CAD build for the part. Positions are in the model's coordinates, mm. A direction names the side the tool comes from. Give positions to 0.01 mm unless a question says otherwise; leave off trailing zeros. Loops run counter-clockwise (first coordinate to the right, second up) from the corner with the lowest first, then second, coordinate; pieces in that order, holes last. Notation, with made-up numbers: M 51,39.25 L 84,39.25 A23 cw 84,67.25 Z; hole C 86,27 d1. An arc over 180 degrees is marked long. One line per question, with ' | ' between items.
```python
from build123d import *

# Parameters (mm, degrees)
SKETCH1_W           = 40.64
SKETCH1_H           = 47.625
SKETCH1_R           = 3.048
BOSS_EXTRUDE1_DEPTH = 6.35
BOSS_EXTRUDE2_DEPTH = 9.906
SKETCH3_R           = 4.826
CUT_EXTRUDE1_DEPTH  = 76.04657711
SKETCH4_R           = 7.1374
CUT_EXTRUDE2_DEPTH  = 9.906
CHAMFER1_SIZE       = 1.5875


with BuildPart() as part:
    # Sketch1 → Boss-Extrude1 (new body)
    with BuildSketch(Plane(origin=(0, 0, 0), x_dir=(1, 0, 0), z_dir=(0, 1, 0))):
        with Locations((20.32, 37.1475)):
            Rectangle(SKETCH1_W, SKETCH1_H)
        with Locations(Location((30.987358569, 18.161641431, 0), (0, 0, 270))):
            Circle(SKETCH1_R, mode=Mode.SUBTRACT)
        with Locations(Location((30.987358569, 43.306358569, 0), (0, 0, 270))):
            Circle(SKETCH1_R, mode=Mode.SUBTRACT)
        with Locations(Location((5.842641431, 18.161641431, 0), (0, 0, 270))):
            Circle(SKETCH1_R, mode=Mode.SUBTRACT)
        with Locations(Location((5.842641431, 43.306358569, 0), (0, 0, 270))):
            Circle(SKETCH1_R, mode=Mode.SUBTRACT)
    extrude(amount=BOSS_EXTRUDE1_DEPTH)

    # Sketch2 → Boss-Extrude2 (add)
    with BuildSketch(Plane(origin=(0, 6.35, 0), x_dir=(1, 0, 0), z_dir=(0, 1, 0))):
        Polygon((31.115, 30.734), (24.765, 41.732522628), (12.065, 41.732522628), (5.715, 30.734), (12.065, 19.735477372), (24.765, 19.735477372), align=None)
    extrude(amount=BOSS_EXTRUDE2_DEPTH)

    # Sketch3 → Cut-Extrude1 (cut, through all)
    with BuildSketch(Plane(origin=(0, 16.256, 0), x_dir=(1, 0, 0), z_dir=(0, 1, 0))):
        with Locations(Location((18.415, 30.734, 0), (0, 0, 270))):
            Circle(SKETCH3_R)
    extrude(amount=-CUT_EXTRUDE1_DEPTH, mode=Mode.SUBTRACT)

    # Sketch4 → Cut-Extrude2 (cut)
    with BuildSketch(Plane(origin=(0, 16.256, 0), x_dir=(1, 0, 0), z_dir=(0, 1, 0))):
        with Locations(Location((18.415, 30.734, 0), (0, 0, 270))):
            Circle(SKETCH4_R)
    extrude(amount=-CUT_EXTRUDE2_DEPTH, mode=Mode.SUBTRACT)

    # Chamfer1
    chamfer1_edges = [part.edges().sort_by_distance(p)[0] for p in [
        (20.32, 6.35, -60.96),
        (0, 6.35, -37.1475),
        (27.94, 16.256, -25.234738686),
        (27.94, 16.256, -36.233261314),
        (18.415, 16.256, -41.732522628),
        (8.89, 16.256, -36.233261314),
        (8.89, 16.256, -25.234738686),
        (18.415, 16.256, -19.735477372),
        (20.32, 6.35, -13.335),
        (40.64, 6.35, -37.1475),
    ]]
    chamfer(chamfer1_edges, length=CHAMFER1_SIZE)


solid = part.part
```
Item 1: Drill centre lines: line 1 along Z through (x, y) = (31, 1.75) (3 decimals); line 2 along Z through (x, y) = (18, 8); line 3 along Z through (x, y) = (4.5, 5.25). Where is each one in solid material? Low to high. Write a range as [from, to].
Conclusion:
line 1: [-60.96, -46.354], [-40.258, -21.21], [-15.114, -13.335] | line 2: [-41.73, -37.86], [-23.61, -19.74] | line 3: [-60.47, -46.04], [-40.57, -20.9], [-15.43, -13.82]
Item 2: 3-axis set-ups, long thin cutter, end or side, ignore diameter. For faces 1 (the flat face through (27.896, 10.451, -25.158)), 2 (the flat face through (8.846, 10.451, -25.312)), 3 (the flat face through (27.98, 10.45, -36.16)), 4 (the flat face through (20, 6.35, -26)), 5 (the flat face through (8.934, 10.451, -36.31)): which of +Z, -Z, +X, -X, +Y, -Y reach the whole face in a straight line?
Conclusion:
face 1: +Z, +X, +Y | face 2: +Z, -X, +Y | face 3: -Z, +X, +Y | face 4: +Y | face 5: -Z, -X, +Y
Item 3: Saw through at D-D on z = -32. Give the cut face in (x, y).
Conclusion:
outline: M 0,0 L 13.76,0 L 13.76,6.35 L 11.39,6.35 L 11.39,16.26 L 8.28,16.26 L 6.45,14.67 L 6.45,6.35 L 1.59,6.35 L 0,4.76 Z; M 23.07,0 L 40.64,0 L 40.64,4.76 L 39.05,6.35 L 30.38,6.35 L 30.38,14.67 L 28.55,16.26 L 25.44,16.26 L 25.44,6.35 L 23.07,6.35 Z
Item 4: Mould opens along X. For faces 6 (the cylindrical face through (34.01, 3.13, -18.56)), 7 (the flat face through (9.63, 15.47, -35.91)), 8 (the flat face through (20, 2, -60.96)) say: pulls with the +X half, pulls with the -X half, needs draft (parallel to the pull), parting line crosses it, or undercut.
Conclusion:
face 6: undercut | face 7: pulls with the -X half | face 8: needs draft
Item 5: Drop flat-ended pins along their axis: P1, Ø5, axis at x = 30.99, z = -18.16, coming from the +Y side; P2, Ø2.5, axis at x = 17.5, y = 12, coming from the +Z side; P3, Ø6.5, axis at x = 20, y = 11, coming from the -Z side; P4, Ø1, axis at x = 4.5, z = -38, coming from the +Y side. Give the stop position or say it passes through.
Conclusion:
P1: through | P2: z = -19.74 | P3: z = -41.73 | P4: y = 6.35
Item 6: Saw through at B-B on z = -53.5. Give the cut face in (x, y).
Conclusion:
outline: M 0,0 L 40.64,0 L 40.64,4.76 L 39.05,6.35 L 1.59,6.35 L 0,4.76 Z
